```python
from build123d import *

# Parameters (mm, degrees)
SKETCH1_W               = 70
SKETCH1_H               = 80
BOSS_EXTRUDE1_DEPTH     = 15
CUT_EXTRUDE1_DEPTH      = 108.354552768
SKETCH3_R               = 3.5
CUT_EXTRUDE2_DEPTH      = 108.354552768
CUT_EXTRUDE3_DEPTH      = 107.77078252
CUT_EXTRUDE3_DEPTH_BACK = 107.77078252
SKETCH4_R               = 3.5
FILLET1_R               = 0.5
FILLET2_R               = 1
CHAMFER1_SIZE           = 1
CHAMFER2_SIZE           = 0.5


with BuildPart() as part:
    # Sketch1 → Boss-Extrude1 (new body)
    with BuildSketch(Plane.XY):
        with Locations((35, 40)):
            Rectangle(SKETCH1_W, SKETCH1_H)
    extrude(amount=BOSS_EXTRUDE1_DEPTH)

    # Sketch2 → Cut-Extrude1 (cut, through all)
    with BuildSketch(Plane.XZ):
        Polygon((18, 15), (8, 5), (62, 5), (52, 15), align=None)
    extrude(amount=-CUT_EXTRUDE1_DEPTH, mode=Mode.SUBTRACT)

    # Sketch3 → Cut-Extrude2 (cut, through all)
    with BuildSketch(Plane.XY.offset(15)):
        with Locations((5, 75)):
            Circle(SKETCH3_R)
    extrude(amount=-CUT_EXTRUDE2_DEPTH, mode=Mode.SUBTRACT)

    # Sketch4 → Cut-Extrude3 (cut, two sides: drawn at the far end of the back side and taken through both)
    with BuildSketch(Plane.XY.offset(5).offset(-CUT_EXTRUDE3_DEPTH_BACK)):
        with Locations((47.5, 17.5)):
            Circle(SKETCH4_R)
    extrude(amount=CUT_EXTRUDE3_DEPTH + CUT_EXTRUDE3_DEPTH_BACK, mode=Mode.SUBTRACT)

    # Fillet1
    # the kernel refuses this fillet: 0.5 mm, written as the material it adds along each edge
    with BuildSketch(Plane(origin=(62, 0, 5), x_dir=(-0.7071067811865527, 0, 0.7071067811865425), z_dir=(0, 1, 0))) as fillet1_piece_1:
        with BuildLine():
            CenterArc((FILLET1_R * 2.41421356237, -FILLET1_R), FILLET1_R, 90, 135)
            Line((FILLET1_R * 1.70710678119, -FILLET1_R * 1.70710678119), (0, 0))
            Line((0, 0), (FILLET1_R * 2.41421356237, 0))
        make_face()
    extrude(amount=80)
    with BuildSketch(Plane(origin=(8, 73.785008685, 5), x_dir=(1, 0, 0), z_dir=(0, 1, 0))) as fillet1_piece_2_section:
        with BuildLine():
            CenterArc((FILLET1_R * 2.41421356237, -FILLET1_R), FILLET1_R, 90, 135)
            Line((FILLET1_R * 1.70710678119, -FILLET1_R * 1.70710678119), (0, 0))
            Line((0, 0), (FILLET1_R * 2.41421356237, 0))
        make_face()
    fillet1_piece_2 = extrude(amount=6.214991315, mode=Mode.PRIVATE)
    fillet1_piece_2 = fillet1_piece_2 - Plane(origin=(5, 75, 5.232830095), x_dir=(1, 0, 0), z_dir=(0, 0, 1)) * Cylinder(3.5, 18, mode=Mode.PRIVATE)
    add(fillet1_piece_2)
    with BuildSketch(Plane(origin=(8, 0, 5), x_dir=(1, 0, 0), z_dir=(0, 1, 0))) as fillet1_piece_3_section:
        with BuildLine():
            CenterArc((FILLET1_R * 2.41421356237, -FILLET1_R), FILLET1_R, 90, 135)
            Line((FILLET1_R * 1.70710678119, -FILLET1_R * 1.70710678119), (0, 0))
            Line((0, 0), (FILLET1_R * 2.41421356237, 0))
        make_face()
    fillet1_piece_3 = extrude(amount=76.214991315, mode=Mode.PRIVATE)
    fillet1_piece_3 = fillet1_piece_3 - Plane(origin=(5, 75, 5.222265381), x_dir=(1, 0, 0), z_dir=(0, 0, 1)) * Cylinder(3.5, 158, mode=Mode.PRIVATE)
    add(fillet1_piece_3)

    # Fillet2
    fillet2_edges = [part.edges().sort_by_distance(p)[0] for p in [
        (18, 40, 15),
        (52, 40, 15),
    ]]
    fillet(fillet2_edges, radius=FILLET2_R)

    # Chamfer1
    chamfer1_edges = [part.edges().sort_by_distance(p)[0] for p in [
        (62.207106781, 80, 15),
        (57.426776695, 0, 9.573223305),
        (57.426776695, 80, 9.573223305),
        (35, 0, 5),
        (35, 80, 5),
        (61.254832985, 0, 5.308658284),
        (61.254832985, 80, 5.308658284),
        (8.745167015, 0, 5.308658284),
        (8.745167015, 80, 5.308658284),
        (62.207106781, 0, 15),
        (12.573223305, 0, 9.573223305),
        (16.50966597, 0, 14.382683432),
        (53.49033403, 0, 14.382683432),
        (7.792893219, 80, 15),
        (12.573223305, 80, 9.573223305),
        (16.50966597, 80, 14.382683432),
        (53.49033403, 80, 14.382683432),
        (7.792893219, 0, 15),
    ]]
    chamfer(chamfer1_edges, length=CHAMFER1_SIZE)

    # Chamfer2
    # the kernel refuses this chamfer: 0.5 mm, written as the material it takes off along each edge
    with BuildSketch(Plane(origin=(5, 75, 0), x_dir=(1, 0, 0), z_dir=(0, -1, 0))) as chamfer2_piece_1:
        Polygon((3.5, CHAMFER2_SIZE), (3.5 + CHAMFER2_SIZE, 0), (3.5, 0), align=None)
    revolve(axis=Axis((5, 75, 0), (0, 0, 1)), mode=Mode.SUBTRACT)
    with BuildSketch(Plane(origin=(5, 75, 15), x_dir=(1, 0, 0), z_dir=(0, -1, 0))) as chamfer2_piece_2:
        Polygon((3.5 + CHAMFER2_SIZE, 0), (3.5, -CHAMFER2_SIZE), (3.5, 0), align=None)
    revolve(axis=Axis((5, 75, 15), (0, 0, 1)), mode=Mode.SUBTRACT)
    with BuildSketch(Plane(origin=(47.5, 17.5, 0), x_dir=(1, 0, 0), z_dir=(0, -1, 0))) as chamfer2_piece_3:
        Polygon((3.5 + CHAMFER2_SIZE, 0), (3.5, CHAMFER2_SIZE), (3.5, 0), align=None)
    revolve(axis=Axis((47.5, 17.5, 0), (0, 0, 1)), mode=Mode.SUBTRACT)
    with BuildSketch(Plane(origin=(47.5, 17.5, 5), x_dir=(1, 0, 0), z_dir=(0, -1, 0))) as chamfer2_piece_4:
        Polygon((3.5 + CHAMFER2_SIZE, 0), (3.5, -CHAMFER2_SIZE), (3.5, 0), align=None)
    revolve(axis=Axis((47.5, 17.5, 5), (0, 0, 1)), mode=Mode.SUBTRACT)


solid = part.part
```
The model under review builds one solid part; all positions refer to its coordinate system, in mm. A direction names the side the tool comes from. Give positions to 0.01 mm unless a question says otherwise; leave off trailing zeros. Write each loop counter-clockwise with the first axis right and the second up, starting at its lowest first coordinate (ties: lowest second). Pieces come first, ordered by that corner, then holes. Notation, with made-up numbers: (65.25, -19) -> (75.25, -19) arc R19 cw to (75.25, 2) -> close; hole circle Ø10 at (27.25, -5). An arc over 180 degrees is marked (long way). Put each result on its own line as item: value.
(1) We need section D-D, the plane y = 75. Give the boundary of the cut face in (x, z).
Results are:
outline: (0, 0) -> (1, 0) -> (1.5, 0.5) -> (1.5, 14.5) -> (1, 15) -> (0, 15) -> close; (8.5, 0.5) -> (9, 0) -> (70, 0) -> (70, 15) -> (54.41, 15) arc R1 ccw to (53.71, 13.29) -> (61.15, 5.85) arc R0.5 cw to (60.79, 5) -> (9.21, 5) arc R0.5 cw to (8.85, 5.85) -> (16.29, 13.29) arc R1 ccw to (15.59, 15) -> (9, 15) -> (8.5, 14.5) -> close
(2) We need section C-C, the plane z = 11.75. Give the boundary of the cut face in (x, y).
Results are:
outline: (0, 0) -> (13.34, 0) -> (14.75, 1) -> (14.75, 79) -> (13.34, 80) -> (0, 80) -> close; (55.25, 1) -> (56.66, 0) -> (70, 0) -> (70, 80) -> (56.66, 80) -> (55.25, 79) -> close; hole circle Ø7 at (5, 75)
(3) We need section B-B, the plane y = 17.5. Give the boundary of the cut face in (x, z).
Results are:
outline: (0, 0) -> (43.5, 0) -> (44, 0.5) -> (44, 4.5) -> (43.5, 5) -> (9.21, 5) arc R0.5 cw to (8.85, 5.85) -> (16.29, 13.29) arc R1 ccw to (15.59, 15) -> (0, 15) -> close; (51, 0.5) -> (51.5, 0) -> (70, 0) -> (70, 15) -> (54.41, 15) arc R1 ccw to (53.71, 13.29) -> (61.15, 5.85) arc R0.5 cw to (60.79, 5) -> (51.5, 5) -> (51, 4.5) -> close
(4) For pin 1 Ø5.5 at (x, y) = (5, 75) entering from +Z; pin 2 Ø15.5 at (x, y) = (28.5, 55) entering from +Z; pin 3 Ø6 at (x, z) = (15, 7.5) entering from -Y, all flat-tipped, find the tip position at first contact; note any pin that passes through.
Results are:
pin 1: through
pin 2: z = 5
pin 3: y = 0.5
(5) We need section A-A, the plane x = 47.5. Give the boundary of the cut face in (y, z), and give its area (4 significant figures).
Results are:
outline: (0, 0) -> (13.5, 0) -> (14, 0.5) -> (14, 4.5) -> (13.5, 5) -> (1, 5) -> (0, 4) -> close; (21, 0.5) -> (21.5, 0) -> (80, 0) -> (80, 4) -> (79, 5) -> (21.5, 5) -> (21, 4.5) -> close
area: 363.5 mm²
(6) To check wall thickness, follow probe 1 along Y at (x, z) = (5, 6.75); probe 2 along X at (y, z) = (29, 13.75); probe 3 along Z at (x, y) = (36, 22.5). State the ranges of each line that lie inside material, in increasing order. Write a range as from..to.
Results are:
probe 1: 0..71.5, 78.5..80
probe 2: 0..16.55, 53.45..70
probe 3: 0..5
(7) Tool access review of faces 4 (the cylindrical face through (16.516, 40.546, 14.367)), 5 (the flat face through (12.28, 79.49, 9.97)), 6 (the flat face through (12.28, 0.51, 9.97)): name each direction out of +Z, -Z, +X, -X, +Y, -Y from which nothing blocks a thin tool from reaching the whole face with its end or side.
Results are:
face 4: +Y, -Y
face 5: +Y
face 6: -Y
(8) The part is to be moulded in two halves that separate along X. For faces 1 (the flat face through (8, 41, 15)), 2 (the cylindrical face through (44.92, 19.865, 2.472)), 3 (the flat face through (0, 39, 7)), say which applies: pulls with the +X half, pulls with the -X half, needs draft (parallel to the pull), parting line crosses it, or undercut.
Results are:
face 1: needs draft
face 2: undercut
face 3: pulls with the -X half
